from build123d import *

# Parameters (mm, degrees)
SKETCH1_W                = 20
SKETCH1_H                = 10
BOSS_EXTRUDE1_DEPTH      = 10
BOSS_EXTRUDE1_DEPTH_BACK = 10
SKETCH3_R                = 2.720672102
BOSS_EXTRUDE2_DEPTH      = 27.695455009
SKETCH6_R                = 2.626203493
BOSS_EXTRUDE3_DEPTH      = 48
SKETCH6_5_W              = 4.878057838
SKETCH6_5_H              = 5.100515908
CUT_EXTRUDE2_DEPTH       = 48
FILLET1_R                = 1
CHAMFER1_SIZE            = 1
FILLET5_R                = 1


with BuildPart() as part:
    # Sketch1 → Boss-Extrude1 (new body, two sides)
    with BuildSketch(Plane.XY) as boss_extrude1_sk:
        with Locations((10, 5)):
            Rectangle(SKETCH1_W, SKETCH1_H)
    extrude(amount=BOSS_EXTRUDE1_DEPTH)
    extrude(boss_extrude1_sk.sketch, amount=-BOSS_EXTRUDE1_DEPTH_BACK)

    # Sketch3 → Boss-Extrude2 (add)
    with BuildSketch(Plane.XY.offset(10)):
        with Locations((10, 5)):
            Circle(SKETCH3_R)
    extrude(amount=BOSS_EXTRUDE2_DEPTH)

    # Sketch6 → Boss-Extrude3 (add)
    with BuildSketch(Plane(origin=(20, 0, 0), x_dir=(0, 0, -1), z_dir=(1, 0, 0))):
        with Locations((-5.764422097, 4.80674108)):
            Circle(SKETCH6_R)
    extrude(amount=BOSS_EXTRUDE3_DEPTH)

    # Sketch6_5 → Cut-Extrude2 (cut)
    with BuildSketch(Plane(origin=(20, 0, 0), x_dir=(0, 0, -1), z_dir=(1, 0, 0))):
        with Locations((4.426041194, 4.399566895)):
            Rectangle(SKETCH6_5_W, SKETCH6_5_H)
    extrude(amount=-CUT_EXTRUDE2_DEPTH, mode=Mode.SUBTRACT)

    # Fillet1
    fillet1_edges = [part.edges().sort_by_distance(p)[0] for p in [
        (7.279327898, 5, 37.695455009),
    ]]
    fillet(fillet1_edges, radius=FILLET1_R)

    # Chamfer1
    chamfer1_edges = [part.edges().sort_by_distance(p)[0] for p in [
        (0, 5, 10),
        (10, 0, 10),
        (20, 5, 10),
        (10, 10, 10),
        (7.279327898, 5, 10),
    ]]
    chamfer(chamfer1_edges, length=CHAMFER1_SIZE)

    # Fillet5
    fillet5_edges = [part.edges().sort_by_distance(p)[0] for p in [
        (68, 4.80674108, 8.390625589),
    ]]
    fillet(fillet5_edges, radius=FILLET5_R)


solid = part.part
Work out the finished part from the listing and answer in its coordinate system (mm). A direction names the side the tool comes from. Round coordinates to 2 decimals unless told otherwise and drop trailing zeros. Write each loop counter-clockwise with the first axis right and the second up, starting at its lowest first coordinate (ties: lowest second). Pieces come first, ordered by that corner, then holes. Notation, with made-up numbers: (78, 4.5) -> (119, 4.5) arc R14 cw to (119, 31.5) -> close; hole circle Ø6 at (-2.5, 72.25). An arc over 180 degrees is marked (long way). Write each question's results on one line, items separated by ' | '.
Item 1: Which of the six approach directions +Z, -Z, +X, -X, +Y, -Y give full straight-line access (tool end or side, diameter ignored) to faces 4 (the face through (10, 6.95, -4)), 5 (the face through (0, 5, 0)), 6 (the face through (10, 10, 0)), 7 (the face through (43.17, 3.21, 7.85)), 8 (the face through (11.26, 2.59, 23.67))?
Result set:
face 4: +X, -X | face 5: +Z, -Z, -X, +Y, -Y | face 6: +Z, -Z, +X, -X, +Y | face 7: +X | face 8: +Z
Item 2: A cutting plane is placed at A-A, the plane x = 10. Determine the outline of the cut face in (y, z).
Result set:
outline: (0, -10) -> (10, -10) -> (10, 9) -> (9, 10) -> (8.72, 10) -> (7.72, 11) -> (7.72, 36.7) arc R1 ccw to (6.72, 37.7) -> (3.28, 37.7) arc R1 ccw to (2.28, 36.7) -> (2.28, 11) -> (1.28, 10) -> (1, 10) -> (0, 9) -> close; hole (1.85, -6.87) -> (6.95, -6.87) -> (6.95, -1.99) -> (1.85, -1.99) -> close
Item 3: The mould has two halves that part along Y. Classify faces 1 (the face through (10, 0, 0)), 2 (the face through (10, 4, -1.987)), 3 (the face through (68, 5, 6)): +Y half, -Y half, draft (parallel to the pull), parting line (faces both ways), or undercut.
Result set:
face 1: -Y half | face 2: undercut | face 3: draft
Item 4: Find the intervals of material crossed by line 1 along Z through (x, y) = (5, 2.75); line 2 along X through (y, z) = (8.75, 4); line 3 along Y through (x, z) = (13, -4), in increasing order. Write a range as [from, to].
Result set:
line 1: [-10, -6.87], [-1.99, 10] | line 2: [0, 20] | line 3: [0, 1.85], [6.95, 10]
Item 5: A cutting plane is placed at B-B, the plane z = 1.5. Determine the outline of the cut face in (x, y), plus the area to 3 significant figures.
Result set:
outline: (0, 0) -> (20, 0) -> (20, 10) -> (0, 10) -> close | area: 200 mm^2
Item 6: Flat-ended cylindrical pins translate along their axes: P1, Ø1.5, axis at x = 13, y = 5, coming from the +Z side; P2, Ø5, axis at x = 59.5, y = 8, coming from the -Z side; P3, Ø1, axis at y = 2.5, z = 15.5, coming from the +X side; P4, Ø2.5, axis at x = 12, y = 6, coming from the +Z side. Find the tip coordinate at first contact, or state that the pin passes through.
Result set:
P1: z = 37.54 | P2: z = 3.23 | P3: x = 11.84 | P4: z = 37.7
Item 7: A cutting plane is placed at D-D, the plane x = 63. Determine the outline of the cut face in (y, z).
Result set:
outline: circle Ø5.25 at (4.81, 5.76)
Item 8: A cutting plane is placed at C-C, the plane z = 33. Determine the outline of the cut face in (x, y), plus the area to 3 significant figures.
Result set:
outline: circle Ø5.44 at (10, 5) | area: 23.3 mm^2
